Model file for the job. Use its own axes, mm. Round coordinates to 2 decimals unless told otherwise and drop trailing zeros. Order: outer loops, then holes, each group sorted by start corner. A loop starts at its lowest first (then second) coordinate and runs counter-clockwise, first axis right, second up. Notation, with made-up numbers: (60.5, 2.25) -> (96.5, 2.25) arc R7 ccw to (96.5, 8.25) -> close; hole circle Ø7 at (72.5, 37). An arc over 180 degrees is marked (long way). Put each result on its own line as item: value. Start each with the question number.
Q1. Pull direction X, two halves, no side cores. Call faces 1 (the face through (-10.4, -10.2, 2.2)), 2 (the face through (-20.4, 20, 2)), 3 (the face through (-11.486, 5.896, 2.218)), 4 (the face through (-10, 40.315, 2)): released by +X, released by -X, zero draft, split by the parting line, or undercut.
Q2. Cut at C-C, the plane z = 2.8. List the corners of the cut face in (x, y).
Q3. Cut at B-B, the plane x = -4. List the corners of the cut face in (y, z).
Q4. Probe L1, parallel to X at y = 2.5, z = 3.7; L2, parallel to Y at x = -5, z = 3.9; L3, parallel to X at y = 35.5, z = 0.9. List the from-to ranges inside material, lowest first.
Q5. Cut at A-A, the plane y = 7. List the corners of the cut face in (x, z), and give its area (3 significant figures).
from build123d import *

# Parameters (mm, degrees)
SKETCH1_R           = 1.5
SKETCH1_R_2         = 1.289902994
BOSS_EXTRUDE1_DEPTH = 4.5


with BuildPart() as part:
    # Sketch1 → Boss-Extrude1 (new body)
    # profile 1 of 3: a face of its own
    with BuildSketch(Plane.XY):
        with BuildLine():
            ThreePointArc((-20.4, 0), (-10.2, 10.2), (0, 0))
            Line((0, 0), (0, 40.315274694))
            Line((0, 40.315274694), (-20.4, 40.315274694))
            Line((-20.4, 40.315274694), (-20.4, 0))
        make_face()
        with Locations((-16.4, 36.315274694)):
            Circle(SKETCH1_R, mode=Mode.SUBTRACT)
        with Locations((-4, 36.315274694)):
            Circle(SKETCH1_R, mode=Mode.SUBTRACT)
    # profile 2 of 3: a face of its own
    with BuildSketch(Plane.XY):
        with BuildLine():
            ThreePointArc((-20.4, 0), (-10.2, -10.2), (0, 0))
            Line((0, 0), (-20.4, 0))
        make_face()
        with Locations((-16.670203746, -2.671416008)):
            Circle(SKETCH1_R, mode=Mode.SUBTRACT)
        with Locations((-7.528583992, -6.470203746)):
            Circle(SKETCH1_R_2, mode=Mode.SUBTRACT)
    # profile 3 of 3: a face of its own
    with BuildSketch(Plane.XY):
        with BuildLine():
            Line((-20.4, 0), (0, 0))
            ThreePointArc((0, 0), (-10.2, 10.2), (-20.4, 0))
        make_face()
        with Locations((-12.871416008, 6.470203746)):
            Circle(SKETCH1_R, mode=Mode.SUBTRACT)
        with Locations((-3.729796254, 2.671416008)):
            Circle(SKETCH1_R, mode=Mode.SUBTRACT)
    extrude(amount=BOSS_EXTRUDE1_DEPTH)


solid = part.part
Ans:
1. face 1: split by the parting line
1. face 2: released by -X
1. face 3: undercut
1. face 4: zero draft
2. outline: (-20.4, 0) arc R10.2 ccw to (0, 0) -> (0, 40.32) -> (-20.4, 40.32) -> close; hole circle Ø3 at (-16.67, -2.67); hole circle Ø3 at (-16.4, 36.32); hole circle Ø3 at (-12.87, 6.47); hole circle Ø2.58 at (-7.53, -6.47); hole circle Ø3 at (-4, 36.32); hole circle Ø3 at (-3.73, 2.67)
3. outline: (-8.1, 0) -> (1.2, 0) -> (1.2, 4.5) -> (-8.1, 4.5) -> close; (4.15, 0) -> (34.82, 0) -> (34.82, 4.5) -> (4.15, 4.5) -> close; (37.82, 0) -> (40.32, 0) -> (40.32, 4.5) -> (37.82, 4.5) -> close
4. L1: x = -20.4 to -5.22, -2.24 to 0
4. L2: y = -8.77 to 1.87, 3.47 to 35.2, 37.43 to 40.32
4. L3: x = -20.4 to -17.66, -15.14 to -5.26, -2.74 to 0
5. outline: (-20.4, 0) -> (-14.27, 0) -> (-14.27, 4.5) -> (-20.4, 4.5) -> close; (-11.47, 0) -> (0, 0) -> (0, 4.5) -> (-11.47, 4.5) -> close
5. area: 79.2 mm^2
